Could you check a few things on this model? Use its own coordinates, in mm. Face numbers are marked on the shaded views. A direction names the side the tool comes from. Round coordinates to 2 decimals unless told otherwise and drop trailing zeros. Loops run counter-clockwise (first coordinate to the right, second up) from the corner with the lowest first, then second, coordinate; pieces in that order, holes last. Notation, with made-up numbers: (46, -5.5) - (58, -5.5) arc R22 cw to (58, 3.5) - close; hole circle Ø2 at (44, -13). An arc over 180 degrees is marked (long way). Answer as CSV lines item,"result". Start each with the question number.
1) Which directions (+Z, -Z, +X, -X, +Y, -Y) give clear straight access to the entire face, cutting with the end or side of a thin tool? Please do the marked faces 1, 2 and 3.
2) Suppose I cut it at B-B, the plane z = 0. Write out the boundary of the cut face in (x, y).
3) We'd pull the mould along Z, two halves only. Please class the marked faces 4, 5 and 6: pulls with the +Z half, pulls with the -Z half, needs draft (parallel to the pull), parting line crosses it, or undercut.
4) Please list where these lines run through material, in increasing order: line 1 along Z through (x, y) = (0, 0.5); line 2 along Y through (x, z) = (0, -3.5); line 3 along Y through (x, z) = (4, -6.25).
5) I'm going to push flat-ended pins straight in: pin 1 Ø3 at (x, y) = (0, -7.3) entering from -Z; pin 2 Ø1.5 at (y, z) = (-5, 4) entering from -X; pin 3 Ø8 at (x, y) = (-6, -7) entering from +Z. Where does each tip first touch, or does it pass through?
6) Suppose I cut it at C-C, the plane x = -6.25. Write out the boundary of the cut face in (y, z), then the cut area to 3 significant figures.
7) Suppose I cut it at A-A, the plane x = 0. Write out the boundary of the cut face in (y, z).
8) Suppose I cut it at D-D, the plane y = 1. Write out the boundary of the cut face in (x, z).
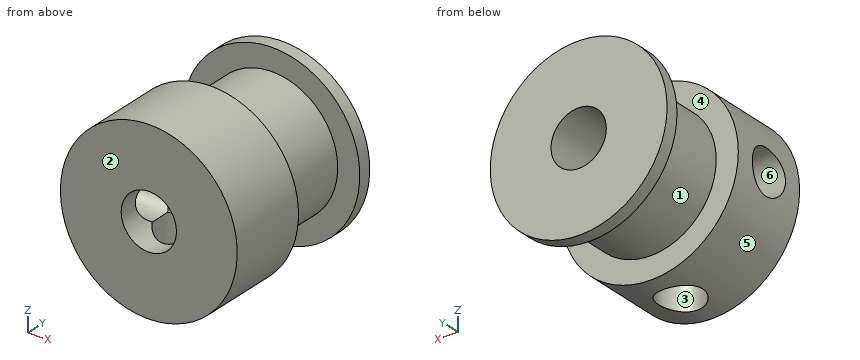
```python
from build123d import *

# Parameters (mm, degrees)
CUT_EXTRUDE1_REACH      = 21.596
SKETCH2_R               = 2.5
CUT_EXTRUDE2_REACH      = 17.78
CUT_EXTRUDE2_END_RADIUS = 8
SKETCH3_R               = 2
CIRPATTERN1_COUNT       = 2
CIRPATTERN1_ANGLE       = 90


with BuildPart() as part:
    # Sketch1 → Revolve1 (revolve)
    with BuildSketch(Plane.XY):
        Polygon((0, 5), (-8, 5), (-8, 3.8), (-6, 3.8), (-6, -3.6), (-8, -3.6), (-8, -11), (0, -11), align=None)
    revolve(axis=Axis((0, 1004.776363636, 0), (0, -1, 0)))

    # Sketch2 → Cut-Extrude1 (cut, up to next)
    with BuildSketch(Plane(origin=(0, 5, 0), x_dir=(1, 0, 0), z_dir=(0, 1, 0)), mode=Mode.PRIVATE) as cut_extrude1_sk1:
        with Locations(Location((0, 0, 0), (0, 0, 180))):
            Circle(SKETCH2_R)
    cut_extrude1_tool1 = extrude(cut_extrude1_sk1.sketch, amount=-CUT_EXTRUDE1_REACH, mode=Mode.PRIVATE) & part.part
    add(cut_extrude1_tool1.solids().sort_by_distance((0, 5, 0))[0], mode=Mode.SUBTRACT)

    # Cut-Extrude2: up to this cylinder (the profile starts inside it)
    cut_extrude2_end = Plane(origin=(0, -7.3, 0), z_dir=(0, 1, 0)) * Cylinder(CUT_EXTRUDE2_END_RADIUS, 52.56, mode=Mode.PRIVATE)
    # Sketch3 → Cut-Extrude2 (cut, up to the surface)
    with BuildSketch(Plane.XY, mode=Mode.PRIVATE) as cut_extrude2_sk1:
        with Locations((0, -7.3)):
            Circle(SKETCH3_R)
    cut_extrude2_tool1 = extrude(cut_extrude2_sk1.sketch, amount=-CUT_EXTRUDE2_REACH, mode=Mode.PRIVATE) & cut_extrude2_end
    cut_extrude2 = cut_extrude2_tool1.solids().sort_by_distance((0, -7.3, 0))[0]
    add(cut_extrude2, mode=Mode.SUBTRACT)

    # CirPattern1: Cut-Extrude2 ×2 about axis
    cirpattern1_axis = Axis((0, -11, 0), (0, 1, 0))
    for i in range(1, CIRPATTERN1_COUNT):
        add(cut_extrude2.rotate(cirpattern1_axis, i * CIRPATTERN1_ANGLE / (CIRPATTERN1_COUNT - 1)), mode=Mode.SUBTRACT)


solid = part.part
```
Filled sheet:
1,face 1,"none"
1,face 2,"+Z, -Z, +X, -X, -Y"
1,face 3,"-Z"
2,outline,"(-8, -11) - (-2.5, -11) - (-2.5, -9.3) - (-8, -9.3) - close; (-8, -5.3) - (-2.5, -5.3) - (-2.5, 5) - (-8, 5) - (-8, 3.8) - (-6, 3.8) - (-6, -3.6) - (-8, -3.6) - close; (2.5, -11) - (8, -11) - (8, -3.6) - (6, -3.6) - (6, 3.8) - (8, 3.8) - (8, 5) - (2.5, 5) - close"
3,face 4,"needs draft"
3,face 5,"parting line crosses it"
3,face 6,"undercut"
4,line 1,"-6 to -2.5, 2.5 to 6"
4,line 2,"-11 to -9.3, -5.3 to 5"
4,line 3,"-11 to -3.6, 3.8 to 5"
5,pin 1,"z = 2"
5,pin 2,"x = -7.31"
5,pin 3,"z = 7.75"
6,outline,"(-11, -4.99) - (-3.6, -4.99) - (-3.6, 4.99) - (-11, 4.99) - close; (3.8, -4.99) - (5, -4.99) - (5, 4.99) - (3.8, 4.99) - close; hole circle Ø4 at (-7.3, 0)"
6,area,"73.3 mm²"
7,outline,"(-11, -8) - (-9.3, -8) - (-9.3, -2.5) - (-11, -2.5) - close; (-11, 2.5) - (5, 2.5) - (5, 8) - (3.8, 8) - (3.8, 6) - (-3.6, 6) - (-3.6, 8) - (-11, 8) - close; (-5.3, -8) - (-3.6, -8) - (-3.6, -6) - (3.8, -6) - (3.8, -8) - (5, -8) - (5, -2.5) - (-5.3, -2.5) - close"
8,outline,"circle Ø12 at (0, 0); hole circle Ø5 at (0, 0)"
